```python
from build123d import *

# Parameters (mm, degrees)
SALIENTE_EXTRUIR1_DEPTH = 150
CROQUIS5_R              = 4.25
SALIENTE_EXTRUIR3_DEPTH = 9
CROQUIS6_R              = 2.5
SALIENTE_EXTRUIR4_DEPTH = 15


with BuildPart() as part:
    # Croquis1 → Saliente-Extruir1 (new body)
    with BuildSketch(Plane(origin=(0, 0, 0), x_dir=(1, 0, 0), z_dir=(0, 1, 0))):
        with BuildLine():
            Line((-2.5, -25), (2.5, -25))
            ThreePointArc((2.5, -25), (16.642135624, -19.142135624), (22.5, -5))
            Line((22.5, -5), (22.5, 5))
            ThreePointArc((22.5, 5), (16.642135624, 19.142135624), (2.5, 25))
            Line((2.5, 25), (-2.5, 25))
            ThreePointArc((-2.5, 25), (-16.642135624, 19.142135624), (-22.5, 5))
            Line((-22.5, 5), (-22.5, -5))
            ThreePointArc((-22.5, -5), (-16.642135624, -19.142135624), (-2.5, -25))
        make_face()
    extrude(amount=SALIENTE_EXTRUIR1_DEPTH)

    # Croquis4 → Revolución-Lámina1 (revolve)
    with BuildSketch(Plane(origin=(0, 0, 0), x_dir=(0, 0, -1), z_dir=(1, 0, 0)), mode=Mode.PRIVATE) as revoluci_n_l_mina1_sk:
        Polygon((-23, 150), (-12, 200), (0, 200), (0, 190), (-3.960859411, 190), (-13.233555333, 147.851382173), align=None)
    revolve(revoluci_n_l_mina1_sk.sketch.rotate(Axis((0, 150, 0), (0, 1, 0)), 180), axis=Axis((0, 150, 0), (0, 1, 0)))

    # Croquis5 → Saliente-Extruir3 (add)
    with BuildSketch(Plane(origin=(0, 200, 0), x_dir=(1, 0, 0), z_dir=(0, 1, 0))):
        with Locations(Location((0, 0, 0), (0, 0, 270))):
            Circle(CROQUIS5_R)
    extrude(amount=SALIENTE_EXTRUIR3_DEPTH)

    # Croquis6 → Saliente-Extruir4 (add)
    with BuildSketch(Plane(origin=(0, 209, 0), x_dir=(1, 0, 0), z_dir=(0, 1, 0))):
        with Locations(Location((0, 0, 0), (0, 0, 270))):
            Circle(CROQUIS6_R)
    extrude(amount=SALIENTE_EXTRUIR4_DEPTH)

    # Croquis7 → Revolución-Lámina4 (revolve)
    with BuildSketch(Plane(origin=(0, 0, 0), x_dir=(0, 0, -1), z_dir=(1, 0, 0))):
        Polygon((-2.5, 224), (-1, 228), (-0.063670822, 227.648876558), (-1.563670822, 223.648876558), align=None)
    revolve(axis=Axis((0, 228, 0), (0, -1, 0)))


solid = part.part
```
Source: CAD feature listing. Evaluate the final solid. Frame: model axes, mm. A direction names the side the tool comes from. Round coordinates to 2 decimals unless told otherwise and drop trailing zeros. Loops run counter-clockwise (first coordinate to the right, second up) from the corner with the lowest first, then second, coordinate; pieces in that order, holes last. Notation, with made-up numbers: M 13,79 L 26,79 A33 cw 26,116 Z; hole C -34.5,83 d6. An arc over 180 degrees is marked long. Put each result on its own line as item: value.
(1) Access query for faces 5 (the face through (-1.8, 150, -23.2)), 6 (the face through (0, 74, -25)), 7 (the face through (-2, 209, 2)), 8 (the face through (-2.53, 169.72, -8.034)). Directions: +Z, -Z, +X, -X, +Y, -Y. A direction counts if a zero-diameter tool reaches every point of the face in a straight line with its end or side. Return the directions, or none.
Solutions:
face 5: -Z, +Y
face 6: -Z, +X, -X, +Y, -Y
face 7: +Y
face 8: none
(2) Ray query, line 1 (X direction, y = 136, z = 4); line 2 (Z direction, x = -7.5, y = 166); line 3 (Z direction, x = -3.5, y = 61). Return the intervals inside material, ascending. Write a range as [from, to].
Solutions:
line 1: [-22.5, 22.5]
line 2: [-17.98, -5.4], [5.4, 17.98]
line 3: [-24.97, 24.97]
(3) Section A-A, the plane y = 91. Return loops of the section in (x, z).
Solutions:
outline: M -22.5,-5 A20 ccw -2.5,-25 L 2.5,-25 A20 ccw 22.5,-5 L 22.5,5 A20 ccw 2.5,25 L -2.5,25 A20 ccw -22.5,5 Z
(4) First-contact query: pin 1 (22.5 mm diameter, centred on x = -2, z = -18.5, fed in from +Y); pin 2 (3 mm diameter, centred on y = 98, z = -0.5, fed in from -X); pin 3 (2 mm diameter, centred on y = 71, z = -5, fed in from +X). Flat tips, straight axial feed; report the tip coordinate or a pass-through.
Solutions:
pin 1: y = 200
pin 2: x = -22.5
pin 3: x = 22.5
(5) Section B-B, the plane y = 179. Return loops of the section in (x, z), and give its area (3 significant figures).
Solutions:
outline: C 0,0 d33.24; hole C 0,0 d12.76
area: 740 mm²
(6) Pull-direction query (X, two-part tool) for faces 1 (the face through (-22.5, 74, 0)), 2 (the face through (1.6, 150, 23.1)), 3 (the face through (0, 190, 0)), 4 (the face through (22.5, 74, 0)); classes: released by +X, released by -X, zero draft, split by the parting line, or undercut.
Solutions:
face 1: released by -X
face 2: zero draft
face 3: undercut
face 4: released by +X
